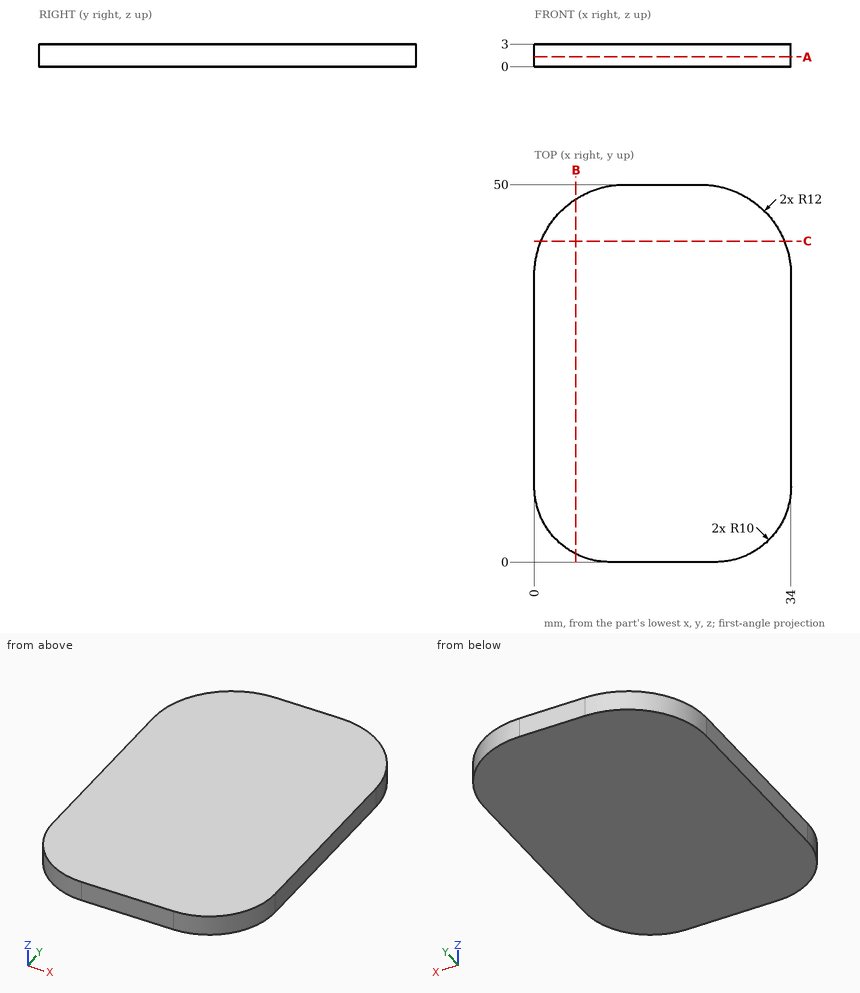
Can you work these out from the drawing? Everything is in mm from the part's minimum corner. Round coordinates to 2 decimals unless told otherwise and drop trailing zeros. Loops run counter-clockwise (first coordinate to the right, second up) from the corner with the lowest first, then second, coordinate; pieces in that order, holes last. Notation, with made-up numbers: M 14.25,89.25 L 43.25,89.25 A22 cw 43.25,105.25 Z; hole C -1.5,70.5 d2. An arc over 180 degrees is marked long. Answer in a Markdown table with one row per item.
1. Please list where these lines run through material, in increasing order: line 1 (X direction, y = 8, z = 2.4); line 2 (Y direction, x = 24, z = 1.5); line 3 (X direction, y = 9.5, z = 2.6). Write a range as from..to.
Established:
| item | result |
|---|---|
| line 1 | 0.2..33.8 |
| line 2 | 0..49.83 |
| line 3 | 0.01..33.99 |
2. If we section it at C-C, the plane y = 42.5: Please give me the cut outline in (x, z), plus the area to 3 significant figures.
Established:
| item | result |
|---|---|
| outline | M 0.88,0 L 33.12,0 L 33.12,3 L 0.88,3 Z |
| area | 96.7 mm² |
3. If we section it at B-B, the plane x = 5.5: Please give me the cut outline in (y, z), plus the area to 3 significant figures.
Established:
| item | result |
|---|---|
| outline | M 1.07,0 L 48.09,0 L 48.09,3 L 1.07,3 Z |
| area | 141 mm² |
4. If we section it at A-A, the plane z = 1.3: Please give me the cut outline in (x, y).
Established:
| item | result |
|---|---|
| outline | M 0,10 A10 ccw 10,0 L 24,0 A10 ccw 34,10 L 34,38 A12 ccw 22,50 L 12,50 A12 ccw 0,38 Z |
